The listing builds one solid part. Answer for the finished solid, in the listing's coordinates (mm). A direction names the side the tool comes from. Round coordinates to 2 decimals unless told otherwise and drop trailing zeros. Loops run counter-clockwise (first coordinate to the right, second up) from the corner with the lowest first, then second, coordinate; pieces in that order, holes last. Notation, with made-up numbers: M 62,-12 L 108,-12 A14 cw 108,10 Z; hole C -24,15 d11. An arc over 180 degrees is marked long. Put each result on its own line as item: value. Start each with the question number.
(1) Which of the six approach directions +Z, -Z, +X, -X, +Y, -Y give full straight-line access (tool end or side, diameter ignored) to faces 5 (the face through (-0.84, 64.86, -38.09)), 6 (the face through (0, 48.895, -37))?
(2) Section A-A, the plane x = 0 is taken. Determine the outline of the cut face in (y, z) (3 decimals), then the cut area to 3 significant figures.
(3) Straight lines are drawn through the part: line 1 (Y direction, x = 34, z = -15) (3 decimals); line 2 (X direction, y = 57, z = -9); line 3 (Z direction, x = 1, y = 9.5). For each, find the intervals that lie inside material, in ascending order.
(4) Flat-ended cylindrical pins translate along their axes: P1, Ø12, axis at y = 10.5, z = -23, coming from the +X side; P2, Ø8, axis at y = 62, z = -4, coming from the -X side; P3, Ø8, axis at y = 46.5, z = -29.5, coming from the +X side; P4, Ø1, axis at y = 43.5, z = -24.5, coming from the -X side. Find the tip coordinate at first contact, or state that the pin passes through.
(5) Section B-B, the plane y = 40 is taken. Determine the outline of the cut face in (x, z), then the cut area to 3 significant figures.
(6) Determine the mould class of faces 1 (the face through (-0.78, 40.74, -35.55)), 2 (the face through (0, 32.385, -37)), 3 (the face through (34, 40, 0)), 4 (the face through (0, 81.28, -30)) for opening direction Y: released by +Y, released by -Y, zero draft, split by the parting line, or undercut.
(7) Section C-C, the plane y = 67 is taken. Determine the outline of the cut face in (x, z).
```python
from build123d import *

# Parameters (mm, degrees)
BOSS_EXTRUDE1_DEPTH = 81.28
SKETCH2_W           = 2.54
SKETCH2_H           = 16.51
CUT_REVOLVE1_ANGLE  = 180
FILLET1_R           = 1.27


with BuildPart() as part:
    # Sketch1 → Boss-Extrude1 (new body)
    with BuildSketch(Plane(origin=(0, 0, 0), x_dir=(1, 0, 0), z_dir=(0, 1, 0))):
        with BuildLine():
            Line((-29.464, 0), (-38.1, 0))
            ThreePointArc((-38.1, 0), (0, 38.1), (38.1, 0))
            Line((38.1, 0), (29.464, 0))
            ThreePointArc((29.464, 0), (0, 29.464), (-29.464, 0))
        make_face()
    extrude(amount=BOSS_EXTRUDE1_DEPTH)

    # Sketch2 → Cut-Revolve1 (revolve, cut)
    with BuildSketch(Plane.XY):
        with Locations((-36.83, 40.64)):
            Rectangle(SKETCH2_W, SKETCH2_H)
    revolve(axis=Axis((0, 0, 0), (0, -1, 0)), revolution_arc=CUT_REVOLVE1_ANGLE, mode=Mode.SUBTRACT)

    # Fillet1
    fillet1_edges = [part.edges().sort_by_distance(p)[0] for p in [
        (0, 48.895, -35.56),
        (0, 32.385, -35.56),
    ]]
    fillet(fillet1_edges, radius=FILLET1_R)


solid = part.part
```
Recorded:
1. face 5: -Z, +Y, -Y
1. face 6: -Z
2. outline: M 0,-38.1 L 32.385,-38.1 L 32.385,-36.83 A1.27 cw 33.655,-35.56 L 47.625,-35.56 A1.27 cw 48.895,-36.83 L 48.895,-38.1 L 81.28,-38.1 L 81.28,-29.464 L 0,-29.464 Z
2. area: 661 mm²
3. line 1: y = 0 to 32.385, 48.895 to 81.28
3. line 2: x = -37.02 to -28.06, 28.06 to 37.02
3. line 3: z = -38.09 to -29.45
4. P1: stops at x = 34.1
4. P2: stops at x = -38.1
4. P3: stops at x = 27.57
4. P4: stops at x = -26.24
5. outline: M -35.56,0 A35.56 ccw 35.56,0 L 29.46,0 A29.46 cw -29.46,0 Z
5. area: 623 mm²
6. face 1: undercut
6. face 2: undercut
6. face 3: zero draft
6. face 4: released by +Y
7. outline: M -38.1,0 A38.1 ccw 38.1,0 L 29.46,0 A29.46 cw -29.46,0 Z
